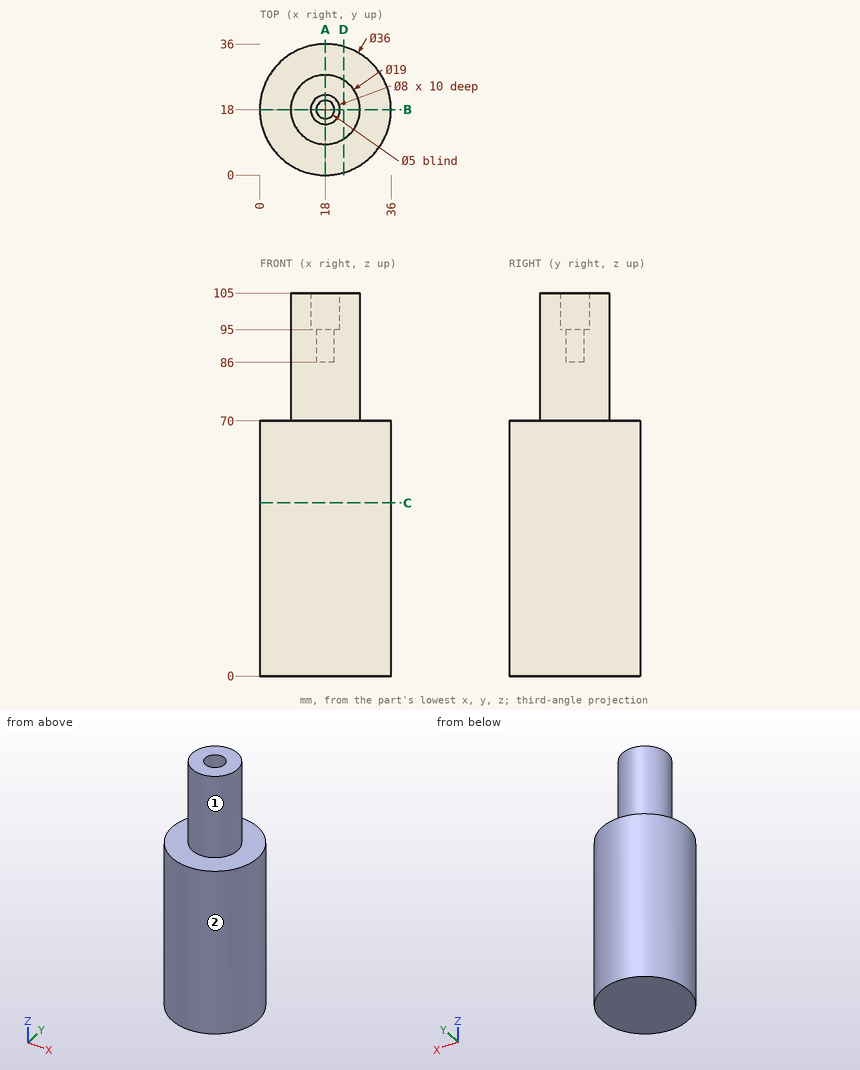
Verification items for this drawing (mm, ordinates from the low corner). A direction names the side the tool comes from. Give positions to 0.01 mm unless a question says otherwise; leave off trailing zeros. Write each loop counter-clockwise with the first axis right and the second up, starting at its lowest first coordinate (ties: lowest second). Pieces come first, ordered by that corner, then holes.
1) Cross-section at A-A (x = 18). Record the boundary of the cut face in (y, z).
Values follow:
outline: (0, 0) - (36, 0) - (36, 70) - (27.5, 70) - (27.5, 105) - (22, 105) - (22, 95) - (20.5, 95) - (20.5, 86) - (15.5, 86) - (15.5, 95) - (14, 95) - (14, 105) - (8.5, 105) - (8.5, 70) - (0, 70) - close
2) Cross-section at C-C (z = 47.5). Record the boundary of the cut face in (x, y).
Values follow:
outline: circle Ø36 at (18, 18)
3) Set-up check for the marked faces 1 and 2: record each of +Z, -Z, +X, -X, +Y, -Y from which the full face is reachable in a straight line by a thin tool's end or side.
Values follow:
face 1: +Z
face 2: +Z, -Z
4) Cross-section at D-D (x = 23). Record the boundary of the cut face in (y, z).
Values follow:
outline: (0.71, 0) - (35.29, 0) - (35.29, 70) - (26.08, 70) - (26.08, 105) - (9.92, 105) - (9.92, 70) - (0.71, 70) - close
5) Go/stop test with flat-tipped pins: pin 1 Ø1 at (y, z) = (16, 89) entering from +X; pin 2 Ø6 at (x, z) = (11, 15) entering from +Y; pin 3 Ø8 at (y, z) = (10.5, 87.5) entering from -X. Record where each tip stops, or that it passes through.
Values follow:
pin 1: stops at x = 27.38
pin 2: stops at y = 35.55
pin 3: stops at x = 9.17
6) Thickness scan on line 1 (Y direction, x = 18, z = 90.5); line 2 (Z direction, x = 31, y = 27); line 3 (X direction, y = 15.5, z = 97). Record the ranges inside material, lowest first.
Values follow:
line 1: y = 8.5 to 15.5, 20.5 to 27.5
line 2: z = 0 to 70
line 3: x = 8.83 to 14.88, 21.12 to 27.17
